Model file for the job. Use its own axes, mm. A direction names the side the tool comes from. Coordinates: 2 decimals unless noted, no trailing zeros. Order: outer loops, then holes, each group sorted by start corner. A loop starts at its lowest first (then second) coordinate and runs counter-clockwise, first axis right, second up.
from build123d import *

# Parameters (mm, degrees)
F0_W      = 130.6576728821
F0_H      = 136.8280164897
F1_DEPTH  = 42.672
F3_DEPTH  = 168.402
F4_W      = 33.3350868896
F4_H      = 81.8327208981
F5_DEPTH  = 7.112
F7_DEPTH  = 20.32
F8_W      = 74.8863741755
F8_H      = 14.6345880348
F9_DEPTH  = 153.162
F10_R     = 8.7751073359
F10_R_2   = 8.9268024196
F10_R_3   = 9.0872621363
F10_R_4   = 9.8396569886
F11_DEPTH = 7.366


with BuildPart() as f1:
    # F0 (on Top) → F1 (new body)
    with BuildSketch(Plane.XY):
        with Locations((2.9565617442, -6.4723659307)):
            Rectangle(F0_W, F0_H)
    extrude(amount=F1_DEPTH)

    # F2 (on face) → F3 (cut)
    with BuildSketch(Plane.YZ.offset(68.2853981853)):
        Polygon((81.023953855, 51.4655448496), (0, 42.672), (83.4134221077, -14.7754913196), align=None)
    extrude(amount=-F3_DEPTH, mode=Mode.SUBTRACT)

    # F4 (on face) → F5 (cut)
    with BuildSketch(Plane.XY.offset(42.672)):
        with Locations((-6.0645765625, -33.9700137265)):
            Rectangle(F4_W, F4_H)
    extrude(amount=-F5_DEPTH, mode=Mode.SUBTRACT)

    # F6 (on face) → F7 (cut)
    with BuildSketch(Plane.YZ.offset(68.2853981853)):
        Polygon((71.3876187801, 35.8445122838), (12.2187227448, 34.2568678656), (12.2187227448, -9.6190823242), (71.3876187801, -9.6190823242), align=None)
    extrude(amount=-F7_DEPTH, mode=Mode.SUBTRACT)

    # F8 (on face) → F9 (cut)
    with BuildSketch(Plane.YZ.offset(68.2853981853)):
        with Locations((-37.4431870878, 4.6425884357)):
            Rectangle(F8_W, F8_H)
    extrude(amount=-F9_DEPTH, mode=Mode.SUBTRACT)

    # F10 (on face) → F11 (cut)
    with BuildSketch(Plane(origin=(0, 19.933646388, 28.943538214), x_dir=(1, 0, 0), z_dir=(0, 0.5672042031, 0.8235771925))):
        with Locations((20.9246538579, 5.7601314038)):
            Circle(F10_R)
        with Locations((-30.0480592996, 5.6009339169)):
            Circle(F10_R_2)
        with Locations((20.8549834788, 39.1954258084)):
            Circle(F10_R_3)
        with Locations((-30.4525401443, 38.9948263764)):
            Circle(F10_R_4)
    extrude(amount=-F11_DEPTH, mode=Mode.SUBTRACT)


solid = f1.part
Q1. Probe line 1 (Z direction, x = -22, y = -25); line 2 (Z direction, x = -29.5, y = -12); line 3 (X direction, y = 18.5, z = 18.5). List the from-to ranges inside material, lowest first.
Established:
line 1: z = 11.96 to 35.56
line 2: z = 11.96 to 42.67
line 3: x = -62.37 to 47.97
Q2. Which spindle directions (+Z, -Z, +X, -X, +Y, -Y) get a long thin tool onto all of the face, cutting with end or side? Do faces 1 (the face through (-6, -33, 35.56)), 2 (the face through (20.728, 45.757, 2.215)), 3 (the face through (4, 0, 6)), 4 (the face through (47.965, 31, 14)). Say none if no direction does.
Established:
face 1: +Z, -Y
face 2: none
face 3: -Z, +X, -X, -Y
face 4: +Z, -Z, +X, +Y
Q3. Mould opens along X. For faces 5 (the face through (-22.732, -35, 39)), 6 (the face through (3.87, 30.54, 21.64)), 7 (the face through (-62.372, -7, 21)) say: pulls with the +X half, pulls with the -X half, needs draft (parallel to the pull), parting line crosses it, or undercut.
Established:
face 5: undercut
face 6: needs draft
face 7: pulls with the -X half
Q4. Cut at B-B, the plane y = -61. List the corners of the cut face in (x, z), plus the area to 3 significant figures.
Established:
outline: (-62.37, 11.96) - (68.29, 11.96) - (68.29, 42.67) - (10.6, 42.67) - (10.6, 35.56) - (-22.73, 35.56) - (-22.73, 42.67) - (-62.37, 42.67) - close
area: 3,780 mm2
Q5. Cut at D-D, the plane y = 42.5. Count the separate pieces of the cut face and the enclosed holes in it, plus the area to 3 significant figures.
Established:
separate pieces: 1
enclosed holes: 2
area: 1,380 mm2
Q6. Drop flat-ended pins along their axis: P1, Ø4, axis at x = 18, y = 43.5, coming from the +Z side; P2, Ø22.5, axis at x = 25, y = -21, coming from the -Z side; P3, Ø0.7, axis at x = 1, z = 37.5, coming from the -Y side. Give the stop position or say it passes through.
Established:
P1: stops at z = 14.09
P2: stops at z = 11.96
P3: stops at y = 6.95
